Can you work these out from the model? Positions are in its coordinate system, mm. Face numbers are marked on the shaded views. A direction names the side the tool comes from. Coordinates: 2 decimals unless noted, no trailing zeros. Loops run counter-clockwise (first coordinate to the right, second up) from the corner with the lowest first, then second, coordinate; pieces in that order, holes last. Notation, with made-up numbers: M 51.25,59.25 L 100.25,59.25 A20 ccw 100.25,75.25 Z; hole C 22.25,56 d6. An arc over 180 degrees is marked long. Return JSON: item names as keys, results as strings. Group by question number.
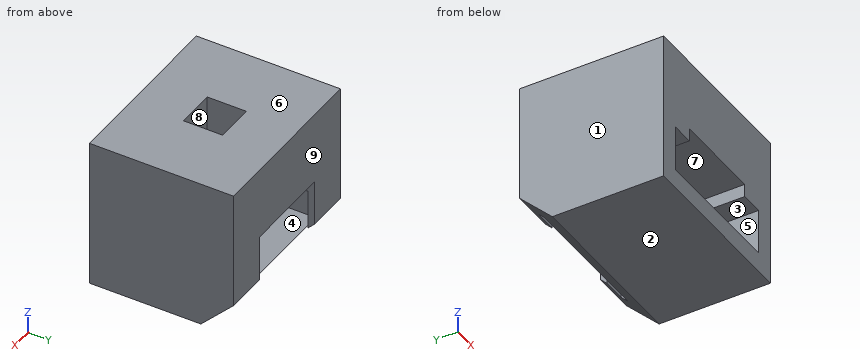
```python
from build123d import *

# Parameters (mm, degrees)
F0_W         = 27
F0_H         = 22
F1_DEPTH     = 20
F2_W         = 21
F2_H         = 21
F3_DEPTH     = 6
F5_DEPTH     = 2
F7_DEPTH     = 20
F8_DEPTH     = 6
F9_W         = 27
F9_H         = 22
F10_DEPTH    = 3
F11_T1_DEPTH = 52.7168298797
F12_DEPTH    = 1


# Not quite as in the source:
# - a fillet or chamfer that OpenCascade refuses, or shapes differently, is made with other operations: its cross-section is extruded or revolved along the edge and cut away or added


with BuildPart() as f1:
    # F0 (on Top) → F1 (new body)
    with BuildSketch(Plane.XY):
        Rectangle(F0_W, F0_H)
    extrude(amount=F1_DEPTH)

    # F2 (on face) → F3 (cut)
    with BuildSketch(Plane(origin=(0, 0, 0), x_dir=(1, 0, 0), z_dir=(0, 0, -1))):
        with Locations((0, 0.5)):
            Rectangle(F2_W, F2_H)
    extrude(amount=-F3_DEPTH, mode=Mode.SUBTRACT)

    # F4 (on face) → F5 (cut)
    with BuildSketch(Plane(origin=(0, 0, 6), x_dir=(1, 0, 0), z_dir=(0, 0, -1))):
        Polygon((0, 11), (-7, 11), (-7, -11), (7, -11), (7, 11), align=None)
    extrude(amount=-F5_DEPTH, mode=Mode.SUBTRACT)

    # F6 (on face) → F7 (cut)
    with BuildSketch(Plane.XY.offset(20)):
        Polygon((0, -3), (3, -3), (3, 3), (-3, 3), (-3, -3), align=None)
    extrude(amount=-F7_DEPTH, mode=Mode.SUBTRACT)

    # F8 (cut): a face of the model
    f8_faces = [f1.faces().sort_by_distance(p)[0] for p in [
        (0, 10.5, 6),
    ]]
    extrude(f8_faces, amount=-F8_DEPTH, mode=Mode.SUBTRACT)

    # F9 (on face) → F10 (join)
    with BuildSketch(Plane(origin=(0, 0, 0), x_dir=(1, 0, 0), z_dir=(0, 0, -1))):
        Rectangle(F9_W, F9_H)
    extrude(amount=F10_DEPTH)

    # F11: chamfer of 5 on 1 edges, made by hand

    # F11_s2 → F11_t1 (cut)
    with BuildSketch(Plane.YZ.offset(-26.3584149398)):
        Polygon((11, 2), (6, -3), (11, -3), align=None)
    extrude(amount=F11_T1_DEPTH, mode=Mode.SUBTRACT)

    # F12 (cut): faces of the model
    f12_faces = [f1.faces().sort_by_distance(p)[0] for p in [
        (8.75, -0.5, 6),
        (-6.7392319038, 0, 8),
        (-8.75, -0.5, 6),
    ]]
    extrude(f12_faces, amount=-F12_DEPTH, mode=Mode.SUBTRACT)


solid = f1.part
```
1) If we mould it in two halves opening along Z, with no side actions, what happens to the marked faces 1, 2, 3 and 4? For each: +Z half, -Z half, draft (parallel to the pull), parting line (faces both ways), or undercut.
2) For pin 1 (6 mm diameter, centred on x = 2, z = 2.5, fed in from +Y); pin 2 (2 mm diameter, centred on x = 5.5, z = 6.5, fed in from +Y); pin 3 (1.8 mm diameter, centred on x = -8, z = 5, fed in from -Y), each with a flat end and sliding along its axis, tell me the tip position at first contact or that it passes through.
3) For the marked faces 5, 6, 7, 8 and 9, which set-ups out of +Z, -Z, +X, -X, +Y, -Y let a thin tool reach every point of the face, with its end or its side?
4) Suppose I cut it at D-D, the plane z = 2.5. List the corners of the cut face in (x, y) for me, then the cut area to 3 significant figures.
5) Suppose I cut it at B-B, the plane y = 7.75. List the corners of the cut face in (x, z) for me.
6) If I drill on line 1 (Z direction, x = 5, y = -2.5); line 2 (X direction, y = 1.75, z = 3); line 3 (Z direction, x = -9, y = 1.75), over which ranges is the centre line in solid material (lowest first)? Write a range as from..to.
7) Suppose I cut it at C-C, the plane x = 9.5. List the corners of the cut face in (y, z) for me.
8) Suppose I cut it at A-A, the plane z = 9.5. List the corners of the cut face in (x, y) for me.
Returned:
{
 "1": {"face 1": "draft", "face 2": "-Z half", "face 3": "undercut", "face 4": "undercut"},
 "2": {"pin 1": "stops at y = 9", "pin 2": "passes through", "pin 3": "stops at y = 10"},
 "3": {"face 5": "-Y", "face 6": "+Z, +X, -X, +Y, -Y", "face 7": "+Y, -Y", "face 8": "+Z", "face 9": "+Z, -Z, +X, -X, +Y"},
 "4": {"outline": "M -13.5,-11 L -10.5,-11 L -10.5,10 L -7,10 L -7,11 L -13.5,11 Z; M 7,10 L 10.5,10 L 10.5,-11 L 13.5,-11 L 13.5,11 L 7,11 Z", "area": "139 mm²"},
 "5": {"outline": "M -13.5,-1.25 L 13.5,-1.25 L 13.5,20 L -13.5,20 Z; hole M -10.5,0 L 10.5,0 L 10.5,7 L 7,7 L 7,9 L -7,9 L -7,7 L -10.5,7 Z"},
 "6": {"line 1": "z = -3..0, 9..20", "line 2": "x = -13.5..-10.5, 10.5..13.5", "line 3": "z = -3..0, 7..20"},
 "7": {"outline": "M -11,-3 L 6,-3 L 9,0 L -11,0 Z; M -11,7 L 10,7 L 10,1 L 11,2 L 11,20 L -11,20 Z"},
 "8": {"outline": "M -13.5,-11 L 13.5,-11 L 13.5,11 L -13.5,11 Z; hole M -3,-3 L 3,-3 L 3,3 L -3,3 Z"}
}
